```python
from build123d import *

# Parameters (mm, degrees)
SKETCH1_R           = 74.295
BOSS_EXTRUDE1_DEPTH = 3.175
SKETCH2_R           = 3.556
SKETCH2_R_2         = 4.191
CUT_EXTRUDE1_DEPTH  = 3.175
SKETCH3_R           = 44.45
CUT_EXTRUDE2_DEPTH  = 3.175


with BuildPart() as part:
    # Sketch1 → Boss-Extrude1 (new body)
    with BuildSketch(Plane(origin=(0, 0, 0), x_dir=(1, 0, 0), z_dir=(0, 1, 0))):
        with Locations(Location((0, 0, 0), (0, 0, 270))):
            Circle(SKETCH1_R)
    extrude(amount=BOSS_EXTRUDE1_DEPTH)

    # Sketch2 → Cut-Extrude1 (cut)
    with BuildSketch(Plane(origin=(0, 3.175, 0), x_dir=(1, 0, 0), z_dir=(0, 1, 0))):
        with Locations(Location((-51.795490029, -24.152633658, 0), (0, 0, 270))):
            Circle(SKETCH2_R)
        with Locations(Location((51.795490029, 24.152633658, 0), (0, 0, 270))):
            Circle(SKETCH2_R)
        with Locations(Location((-53.975, 0, 0), (0, 0, 270))):
            Circle(SKETCH2_R_2)
        with Locations(Location((53.975, 0, 0), (0, 0, 270))):
            Circle(SKETCH2_R_2)
    extrude(amount=-CUT_EXTRUDE1_DEPTH, mode=Mode.SUBTRACT)

    # Sketch3 → Cut-Extrude2 (cut)
    with BuildSketch(Plane(origin=(0, 3.175, 0), x_dir=(1, 0, 0), z_dir=(0, 1, 0))):
        with Locations(Location((0, 0, 0), (0, 0, 270))):
            Circle(SKETCH3_R)
    extrude(amount=-CUT_EXTRUDE2_DEPTH, mode=Mode.SUBTRACT)


solid = part.part
```
Can you work these out from the model? Positions are in its coordinate system, mm. Round coordinates to 2 decimals unless told otherwise and drop trailing zeros. Loops run counter-clockwise (first coordinate to the right, second up) from the corner with the lowest first, then second, coordinate; pieces in that order, holes last. Notation, with made-up numbers: M 12,33 L 70,33 A11 cw 70,41 Z; hole C -6.75,57 d4. An arc over 180 degrees is marked long. Answer in a Markdown table with one row per item.
1. Please list where these lines run through material, in increasing order: line 1 (X direction, y = 1.25, z = 0) (3 decimals); line 2 (X direction, y = 0.8, z = -2); line 3 (X direction, y = 2.75, z = -21). Write a range as from..to.
Established:
| item | result |
|---|---|
| line 1 | -74.295..-58.166, -49.784..-44.45, 44.45..49.784, 58.166..74.295 |
| line 2 | -74.27..-57.66, -50.29..-44.4, 44.4..50.29, 57.66..74.27 |
| line 3 | -71.27..-39.18, 39.18..50.15, 53.44..71.27 |
2. Thinking about a two-plate mould opening in X: for faces 1 (the face through (73.663, 1.565, -9.672)), 2 (the face through (37.48, 1.61, 23.9)), 3 (the face through (-32, 0, 32)), which applies, pulls with the +X half, pulls with the -X half, needs draft (parallel to the pull), parting line crosses it, or undercut?
Established:
| item | result |
|---|---|
| face 1 | parting line crosses it |
| face 2 | undercut |
| face 3 | needs draft |
3. I'm going to push flat-ended pins straight in: pin 1 Ø6 at (x, z) = (52, 53.5) entering from -Y; pin 2 Ø1 at (x, y) = (-55.5, 1.5) entering from +Z. Where does each tip first touch, or does it pass through?
Established:
| item | result |
|---|---|
| pin 1 | y = 0 |
| pin 2 | z = 49.95 |
4. If we section it at B-B, the plane z = 0: Please give me the cut outline in (x, y) (3 decimals), plus the area to 3 significant figures.
Established:
| item | result |
|---|---|
| outline | M -74.295,0 L -58.166,0 L -58.166,3.175 L -74.295,3.175 Z; M -49.784,0 L -44.45,0 L -44.45,3.175 L -49.784,3.175 Z; M 44.45,0 L 49.784,0 L 49.784,3.175 L 44.45,3.175 Z; M 58.166,0 L 74.295,0 L 74.295,3.175 L 58.166,3.175 Z |
| area | 136 mm² |
5. If we section it at A-A, the plane x = 0: Please give me the cut outline in (y, z) (3 decimals), plus the area to 3 significant figures.
Established:
| item | result |
|---|---|
| outline | M 0,-74.295 L 3.175,-74.295 L 3.175,-44.45 L 0,-44.45 Z; M 0,44.45 L 3.175,44.45 L 3.175,74.295 L 0,74.295 Z |
| area | 190 mm² |
6. If we section it at D-D, the plane z = 23: Please give me the cut outline in (x, y) (1 decimal).
Established:
| item | result |
|---|---|
| outline | M -70.6,0 L -55.2,0 L -55.2,3.2 L -70.6,3.2 Z; M -48.4,0 L -38,0 L -38,3.2 L -48.4,3.2 Z; M 38,0 L 70.6,0 L 70.6,3.2 L 38,3.2 Z |
7. If we section it at C-C, the plane z = -34: Please give me the cut outline in (x, y) (3 decimals), plus the area to 3 significant figures.
Established:
| item | result |
|---|---|
| outline | M -66.059,0 L -28.632,0 L -28.632,3.175 L -66.059,3.175 Z; M 28.632,0 L 66.059,0 L 66.059,3.175 L 28.632,3.175 Z |
| area | 238 mm² |
